from build123d import *

# Parameters (mm, degrees)
SKETCH1_R           = 30
BOSS_EXTRUDE1_DEPTH = 30
CUT_EXTRUDE1_DEPTH  = 10


with BuildPart() as part:
    # Sketch1 → Boss-Extrude1 (new body)
    with BuildSketch(Plane(origin=(0, 0, 0), x_dir=(0, 0, -1), z_dir=(1, 0, 0))):
        Circle(SKETCH1_R)
    extrude(amount=BOSS_EXTRUDE1_DEPTH)

    # Sketch2 → Cut-Extrude1 (cut)
    with BuildSketch(Plane.ZY):
        Polygon((3.050745315, -2.135521721), (3.374788718, 1.574262083), (0.324043403, 3.709783804), (-3.050745315, 2.135521721), (-3.374788718, -1.574262083), (-0.324043403, -3.709783804), align=None)
    extrude(amount=-CUT_EXTRUDE1_DEPTH, mode=Mode.SUBTRACT)


solid = part.part
Design review of the part built by this model. Coordinates are the model's own, in mm. A direction names the side the tool comes from. Coordinates: 2 decimals unless noted, no trailing zeros. Loops run counter-clockwise (first coordinate to the right, second up) from the corner with the lowest first, then second, coordinate; pieces in that order, holes last.
Item 1: Wall thickness on L1, parallel to Y at x = 9.5, z = 2; L2, parallel to Z at x = 18.5, y = 19.5; L3, parallel to Z at x = 18.75, y = 10: over which ranges is each line inside the solid? List them lowest first.
Completed:
L1: y = -29.93 to -2.63, 2.54 to 29.93
L2: z = -22.8 to 22.8
L3: z = -28.28 to 28.28
Item 2: Add section B-B (y = 0). Write out the cut boundary in (x, z), and give its area (3 significant figures).
Completed:
outline: (0, -30) - (30, -30) - (30, 30) - (0, 30) - (0, 3.24) - (10, 3.24) - (10, -3.24) - (0, -3.24) - close
area: 1,740 mm2
Item 3: Add section A-A (x = 2.75). Write out the cut boundary in (y, z).
Completed:
outline: circle Ø60 at (0, 0); hole (-3.71, -0.32) - (-1.57, -3.37) - (2.14, -3.05) - (3.71, 0.32) - (1.57, 3.37) - (-2.14, 3.05) - close
Item 4: Draft analysis for pull direction Y (two halves, no side actions). For faces 1 (the cylindrical face through (14.79, 1.32, 29.97)), 2 (the flat face through (4.93, 2.934, -1.34)), 3 (the flat face through (0, 0, -6)), state which applies: pulls with the +Y half, pulls with the -Y half, needs draft (parallel to the pull), parting line crosses it, or undercut.
Completed:
face 1: parting line crosses it
face 2: undercut
face 3: needs draft
Item 5: Clearance check with flat-ended pins moving along their axes: pin 1 (8 mm diameter, centred on x = 11, y = 13.5, fed in from +Z); pin 2 (12 mm diameter, centred on y = 23, z = 22, fed in from +X); pin 3 (3 mm diameter, centred on x = 15, y = -3, fed in from +Z); pin 4 (8 mm diameter, centred on x = 12.5, z = -13, fed in from +Y). State where each tip first meets the part, or that it passes through.
Completed:
pin 1: stops at z = 28.46
pin 2: stops at x = 30
pin 3: stops at z = 29.96
pin 4: stops at y = 28.62
Item 6: Add section D-D (z = -26). Write out the cut boundary in (x, y).
Completed:
outline: (0, -14.97) - (30, -14.97) - (30, 14.97) - (0, 14.97) - close
Item 7: Add section C-C (x = 20.25). Write out the cut boundary in (y, z), and give its area (3 significant figures).
Completed:
outline: circle Ø60 at (0, 0)
area: 2,830 mm2
Item 8: For faces 4 (the flat face through (30, 0, 0)), 5 (the flat face through (4.93, 0.31, -3.21)), list the 3-axis set-ups (+Z, -Z, +X, -X, +Y, -Y) from which the entire face can be reached by the end or side of a thin tool; tool diameter is ignored.
Completed:
face 4: +Z, -Z, +X, +Y, -Y
face 5: -X
